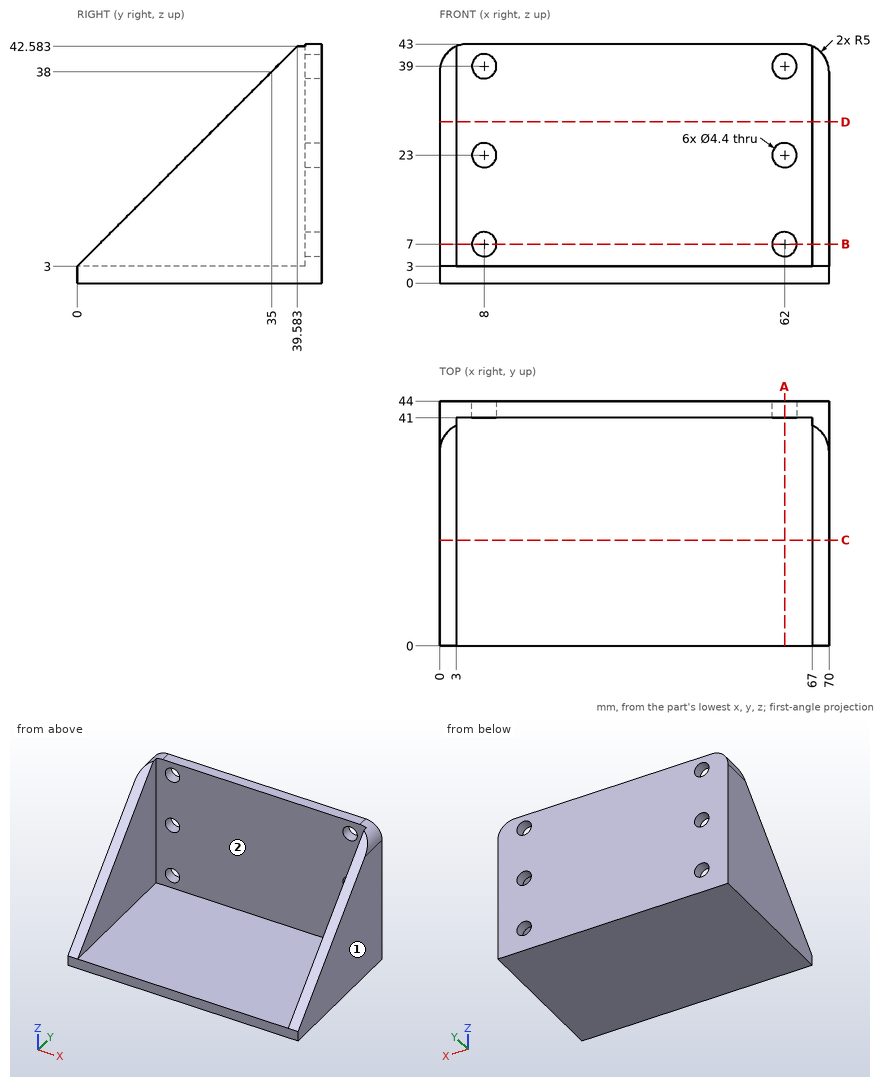
Part print with two shaded views. Sizes in mm from the minimum x, y, z corner. A direction names the side the tool comes from. Round coordinates to 2 decimals unless told otherwise and drop trailing zeros. Loops run counter-clockwise (first coordinate to the right, second up) from the corner with the lowest first, then second, coordinate; pieces in that order, holes last.
1. Drill centre lines: line 1 along Z through (x, y) = (62, 41.95); line 2 along X through (y, z) = (39, 13); line 3 along Y through (x, z) = (36.5, 20). Where is each one in solid material? Low to high.
Solutions:
line 1: z = 0 to 4.8, 9.2 to 20.8, 25.2 to 36.8, 41.2 to 43
line 2: x = 0 to 3, 67 to 70
line 3: y = 41 to 44
2. Slice it at C-C (y = 19). Give the cut face in (x, z).
Solutions:
outline: (0, 0) - (70, 0) - (70, 22) - (67, 22) - (67, 3) - (3, 3) - (3, 22) - (0, 22) - close
3. 3-axis set-ups, long thin cutter, end or side, ignore diameter. For the marked faces 1 and 2: which of +Z, -Z, +X, -X, +Y, -Y reach the whole face in a straight line?
Solutions:
face 1: +Z, -Z, +X, +Y, -Y
face 2: +Z, -Y
4. Slice it at A-A (x = 62). Give the cut face in (y, z).
Solutions:
outline: (0, 0) - (44, 0) - (44, 4.8) - (41, 4.8) - (41, 3) - (0, 3) - close; (41, 9.2) - (44, 9.2) - (44, 20.8) - (41, 20.8) - close; (41, 25.2) - (44, 25.2) - (44, 36.8) - (41, 36.8) - close; (41, 41.2) - (44, 41.2) - (44, 43) - (41, 43) - close
5. Flat gauge pins, fed straight in: pin 1 (5 mm diameter, centred on x = 9.5, y = 5.5, fed in from +Z); pin 2 (12 mm diameter, centred on y = 13, z = 20, fed in from +X); pin 3 (2.5 mm diameter, centred on x = 62, z = 7, fed in from -Y); pin 4 (20 mm diameter, centred on x = 41.5, z = 30, fed in from -Y). Where does each tip first touch, or does it go through?
Solutions:
pin 1: stops at z = 3
pin 2: stops at x = 70
pin 3: passes through
pin 4: stops at y = 41
6. Slice it at D-D (z = 29). Give the cut face in (x, y), and give its area (3 significant figures).
Solutions:
outline: (0, 26) - (3, 26) - (3, 41) - (67, 41) - (67, 26) - (70, 26) - (70, 44) - (0, 44) - close
area: 300 mm2
7. Slice it at B-B (z = 7). Give the cut face in (x, y).
Solutions:
outline: (0, 4) - (3, 4) - (3, 41) - (5.8, 41) - (5.8, 44) - (0, 44) - close; (10.2, 41) - (59.8, 41) - (59.8, 44) - (10.2, 44) - close; (64.2, 41) - (67, 41) - (67, 4) - (70, 4) - (70, 44) - (64.2, 44) - close
